Autodesk Inventor part; units mm, degrees
ref_plane "Płaszczyzna konstrukcyjna1" through (-150, 3.5, 2) normal (0, -1, 0) x (1, 0, 0)
ref_plane "YZ Plane" through (0, 0, 0) normal (1, 0, 0) x (0, 1, 0)
ref_plane "XZ Plane" through (0, 0, 0) normal (0, 1, 0) x (-1, 0, 0)
sketch "Szkic1" plane through (-150, 0, 2) normal (0, -1, 0) x (1, 0, 0)
  circle A0 centre (150, -2) radius 2.4
  line L0 (150, -2) -> (150, 8)
  line L1 (150, -2) -> (150, -12)
  arc A1 (150, -12) -> (150, 8) centre (150, -2) ccw
  line L2 (150, -2) -> (0, -2)
  line L3 (150, -2) -> (300, -2) construction
  line L4 (0, -2) -> (0, 0)
  line L5 (0, -2) -> (0, -4)
  line L6 (0, -4) -> (150, -12)
  line L7 (0, 0) -> (150, 8)
  dimension "d0" = 4.8
  dimension "d1" = 10
  dimension "d2" = 10
  dimension "d3" = 150
  dimension "d4" = 180
  dimension "d5" = 2
  dimension "d6" = 2
extrude "Wyciągnięcie proste1" add sketch "Szkic1" against normal blind 8 contours A0 L0 A1 L1 | A0 L2 L4 L7 L0 | L1 L6 L5 L2 A0
sketch "Szkic2" plane through (-150, 8, 2) normal (0, 1, 0) x (1, 0, 0)
  circle A0 centre (150, 2) radius 2.4
  circle A1 centre (150, 2) radius 2.95
  dimension "d9" = 5.9
extrude "Wyciągnięcie proste2" cut sketch "Szkic2" against normal blind 4
ref_plane "Płaszczyzna konstrukcyjna1" through (-150, 3.5, 2) normal (0, -1, 0) x (1, 0, 0)
sketch "Szkic4" plane through (-150, 3.5, 2) normal (0, -1, 0) x (1, 0, 0)
  circle A0 centre (150, -2) radius 1.5
  circle A1 centre (150, -2) radius 2.4
  dimension "d13" = 3
extrude "Wyciągnięcie proste3" add sketch "Szkic4" along normal blind 1
sketch "Szkic5" plane through (-150, 8, 2) normal (0, 1, 0) x (1, 0, 0)
  line L0 (129.6292, 9.8056) -> (142.004, 9.8056) construction
  line L1 (142.004, 9.8056) -> (142.004, -5.0441) construction
  line L2 (142.004, -5.0441) -> (129.6292, -5.0441) construction
  line L3 (129.6292, -5.0441) -> (129.6292, 9.8056) construction
  point P0 (150, 2)
sketch "Szkic6" plane through (-150, 8, 2) normal (0, 1, 0) x (1, 0, 0)
  circle A0 centre (150, 2) radius 1.5
  line L0 (150, 2) -> (0, 2)
  line L1 (150, 2) -> (300, 2) construction
  line L2 (0, 2) -> (5.6, 2)
  line L3 (5.6, 2) -> (-16.8, 2)
  line L4 (5.6, 2) -> (-16.8, 2)
  line L5 (-16.8, 2) -> (-16.8, -4.5)
  line L6 (-16.8, -4.5) -> (5.6, -4.5)
  line L7 (5.6, -4.5) -> (5.6, 2)
  line L8 (5.6, 2) -> (-16.8, 2)
  line L9 (-16.8, 2) -> (-16.8, 8.5)
  line L10 (-16.8, 8.5) -> (5.6, 8.5)
  line L11 (5.6, 8.5) -> (5.6, 2)
  line L12 (5.6, 8.5) -> (5.6, 9.5)
  line L13 (5.6, 9.5) -> (6.6, 9.5)
  line L14 (-16.8, -4.5) -> (-16.8, -5.5)
  line L15 (-16.8, -5.5) -> (-17.8, -5.5)
  line L16 (-17.8, -5.5) -> (6.6, -5.5)
  line L17 (6.6, -5.5) -> (6.6, 9.5)
  line L18 (6.6, 9.5) -> (-17.8, 9.5)
  line L19 (-17.8, 9.5) -> (-17.8, -5.5)
  line L20 (6.6, -5.5) -> (14.7626, -0.7873)
  line L21 (150, -8) -> (0, 0)
  line L22 (6.6, -5.5) -> (16.0253, -5.5) construction
  line L23 (6.6, 9.5) -> (14.7626, 4.7873)
  line L24 (14.7626, -0.7873) -> (14.7626, 4.7873)
  point P0 (5.6, 9.5)
  dimension "d16" = 150
  dimension "d17" = 180
  dimension "d18" = 5.6
  dimension "d19" = 22.4
  dimension "d20" = 6.5
  dimension "d21" = 6.5
  dimension "d22" = 1
  dimension "d23" = 1
  dimension "d24" = 1
  dimension "d25" = 1
  dimension "d26" = 30
extrude "Wyciągnięcie proste4" add sketch "Szkic6" along normal blind 8 contours L11 L12 L13 L17 L0 | L0 L17 L21 L7 | L17 L23 L24 L0 | L0 L24 L21 L17 | L21 L17 L16 L14 L6 L7 | L10 L9 L5 L14 L15 L19 L18 L12 | L21 L20 L17
sketch "Szkic7" plane through (-150, 8, 2) normal (0, 1, 0) x (1, 0, 0)
  circle A0 centre (150, 2) radius 1.5
  line L0 (150, 2) -> (140, 2)
  line L1 (140, 2) -> (140, -5)
  line L2 (140, 2) -> (140, 9)
  line L3 (140, 2) -> (40, 2)
  line L4 (40, 2) -> (140, 9)
  line L5 (40, 2) -> (140, -5)
  line L6 (5.6, -0.2987) -> (5.6, 4.2987)
  line L7 (5.6, 4.2987) -> (5.6, -0.2987)
  line L8 (0, 0) -> (5.6, -0.2987)
  line L9 (5.6, -0.2987) -> (0, 0)
  line L10 (0, 0) -> (0, 4.0412)
  line L11 (0, 4.0412) -> (5.6, 4.2987)
  dimension "d29" = 10
  dimension "d30" = 7
  dimension "d31" = 7
  dimension "d32" = 100
extrude "Wyciągnięcie proste5" cut sketch "Szkic7" against normal through all contours L3 L4 L2 | L1 L5 L3 | L8 L10 L11 L6
chamfer "Faza1" distance 8 angle 45 1 edges at (-135.2374, 8, 0)
chamfer "Faza2" distance 8 angle 45 1 edges at (-144.4, 0, 0)
sketch "Szkic8" plane through (-150, 0, 2) normal (0, -1, 0) x (1, 0, 0)
  circle A0 centre (150, -2) radius 2.4
  line L0 (150, -2) -> (0, -2)
  circle A1 centre (0, -2) radius 2
  dimension "d41" = 150
  dimension "d42" = 4
sketch "Szkic9" plane through (-150, 8, 2) normal (0, -1, 0) x (1, 0, 0)
  point P0 (150, -2)
sketch "Szkic10" plane through (-150, 0, 2) normal (0, -1, 0) x (1, 0, 0)
  circle A0 centre (150, -2) radius 2.85
  dimension "d43" = 5.7
extrude "Wyciągnięcie proste6" cut sketch "Szkic10" against normal blind 2.5
properties part number "pointrer"
The model under review builds one solid part; all positions refer to its coordinate system, in mm. A direction names the side the tool comes from. Round coordinates to 2 decimals unless told otherwise and drop trailing zeros. Order: outer loops, then holes, each group sorted by start corner. A loop starts at its lowest first (then second) coordinate and runs counter-clockwise, first axis right, second up. Notation, with made-up numbers: (11, 70.5) - (26, 70.5) arc R18 cw to (26, 90.5) - close; hole circle Ø1 at (46.25, -16). An arc over 180 degrees is marked (long way). Answer in a Markdown table with one row per item.
(1) Mouldability with a two-part tool opening along X and no side actions: class faces 1 (the face through (-156, 12, 6.5)), 2 (the face through (-155, 12, 7.5)), 3 (the face through (10, 4, 0)) as released by +X, released by -X, zero draft, split by the parting line, or undercut.
Result set:
| item | result |
|---|---|
| face 1 | undercut |
| face 2 | zero draft |
| face 3 | released by +X |
(2) Machinability: for faces 4 (the face through (-2.262, 1.232, -1.734)), 5 (the face through (0, 3.5, -2)), 6 (the face through (-156, 12, -6.5)), which of the approach directions +Z, -Z, +X, -X, +Y, -Y give a long, thin tool a straight path to every point of the face, cutting with its end or side? Answer none if there is none.
Result set:
| item | result |
|---|---|
| face 4 | -Y |
| face 5 | +Y |
| face 6 | +Y, -Y |
(3) Take a section at C-C on x = -93. Write out the cut boundary in (y, z).
Result set:
| item | result |
|---|---|
| outline | (0, -5.04) - (8, -5.04) - (8, -1.19) - (0, -1.19) - close; (0, 1.19) - (8, 1.19) - (8, 5.04) - (0, 5.04) - close |
(4) For line 1 (Z direction, x = 0, y = 2.95); line 2 (Z direction, x = -158, y = 10); line 3 (Y direction, x = -6.5, z = -6.25), list the stretches that pass through material, from the lowest coordinate up. Write a range as from..to.
Result set:
| item | result |
|---|---|
| line 1 | z = -10..-1.5, 1.5..10 |
| line 2 | z = -7.5..-6.5, 6.5..7.5 |
| line 3 | y = 0..8 |
(5) Take a section at A-A on x = -146. Write out the cut boundary in (y, z), plus the area to 3 significant figures.
Result set:
| item | result |
|---|---|
| outline | (8, -7.5) - (16, -7.5) - (16, -6.5) - (8, -6.5) - close; (8, 6.5) - (16, 6.5) - (16, 7.5) - (8, 7.5) - close |
| area | 16.0 mm2 |
(6) Clearance check with flat-ended pins moving along their axes: P1, Ø9, axis at x = -158.5, y = 13.5, coming from the -Z side; P2, Ø1.5, axis at y = 9, z = 6.5, coming from the +X side; P3, Ø8, axis at x = -101, z = -6.5, coming from the -Y side; P4, Ø1.4, axis at x = 1, z = 0.5, coming from the +Y side. State where each tip first meets the part, or that it passes through.
Result set:
| item | result |
|---|---|
| P1 | stops at z = -7.5 |
| P2 | stops at x = -140.37 |
| P3 | stops at y = 0 |
| P4 | stops at y = 3.5 |
